For this review, take the finished solid that the model builds, in its own axes (mm). Face numbers are marked on the shaded views. A direction names the side the tool comes from. Coordinates: 2 decimals unless noted, no trailing zeros. Loops run counter-clockwise (first coordinate to the right, second up) from the corner with the lowest first, then second, coordinate; pieces in that order, holes last. Notation, with made-up numbers: (19, 71.5) - (45, 71.5) arc R25 cw to (45, 94.5) - close; hole circle Ø11 at (51, 88.5). An arc over 180 degrees is marked (long way). One line per item, written item: value. Start each with the question number.
1. The part is to be moulded in two halves that separate along X. For the marked faces 3, 4, 5 and 6, say which applies: released by +X, released by -X, zero draft, split by the parting line, or undercut.
2. Insertion check: pin 1 (5.5 mm diameter, centred on x = 0, z = -14, fed in from -Y). The pin has a flat end and moves straight along its axis. Give the tip position at first contact, or say it passes through.
3. To check wall thickness, follow line 1 (Z direction, x = 0, y = 19); line 2 (X direction, y = 21.75, z = 4); line 3 (X direction, y = 10, z = -14). State the ranges of each line that lie inside material, in increasing order. Write a range as from..to.
4. Take a section at B-B, the plane z = -14. State the section outline as (x, y) points, and give its area (3 significant figures).
5. Take a section at D-D, the plane x = 0. State the section outline as (y, z) points, and give its area (3 significant figures).
6. For the marked faces 1 and 2, list the 3-axis set-ups (+Z, -Z, +X, -X, +Y, -Y) from which the entire face can be reached by the end or side of a thin tool; tool diameter is ignored.
7. Take a section at A-A, the plane x = 4.5. State the section outline as (y, z) points.
8. Take a section at C-C, the plane y = 14.5. State the section outline as (x, z) points, and give its area (3 significant figures).
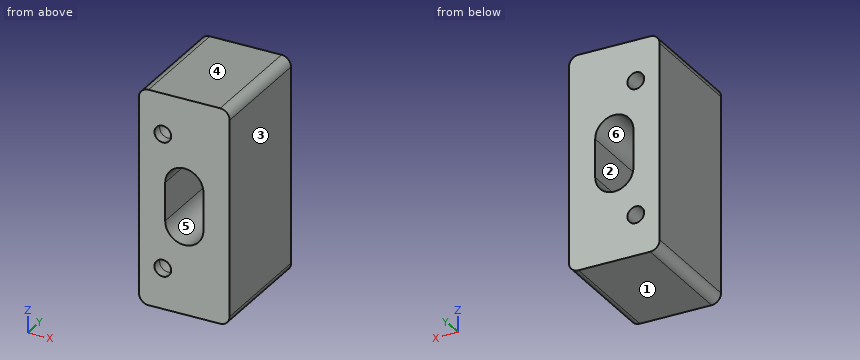
```python
from build123d import *
from build123d.topology import SkipClean

# Parameters (mm, degrees)
SKETCH_1_W          = 19
SKETCH_1_H          = 45
SKETCH_1_R          = 1.75
EXTRUDE_1_DEPTH     = 2
FILLET_1_R          = 2
CUT_EXTRUDE_1_DEPTH = 2
EXTRUDE_START       = 21.612698372
SKETCH_4_R          = 1.75
EXTRUDE_2_DEPTH     = 21.612698372


with BuildPart() as part:
    # 草图1 → 凸台-拉伸1 (new body)
    with BuildSketch(Plane(origin=(0, 0, 0), x_dir=(1, 0, 0), z_dir=(0, 1, 0))):
        with Locations((4.5, 0)):
            Rectangle(SKETCH_1_W, SKETCH_1_H)
        with Locations(Location((0, -14, 0), (0, 0, 270))):
            Circle(SKETCH_1_R, mode=Mode.SUBTRACT)
        with Locations(Location((0, 14, 0), (0, 0, 270))):
            Circle(SKETCH_1_R, mode=Mode.SUBTRACT)
    extrude(amount=EXTRUDE_1_DEPTH)

    # 圆角1
    fillet_1_edges = [part.edges().sort_by_distance(p)[0] for p in [
        (-5, 1, -22.5),
        (14, 1, -22.5),
        (14, 1, 22.5),
        (-5, 1, 22.5),
    ]]
    fillet(fillet_1_edges, radius=FILLET_1_R)

    # 草图3 → 切除-拉伸1 (cut)
    with BuildSketch(Plane(origin=(0, 2, 0), x_dir=(1, 0, 0), z_dir=(0, 1, 0))):
        with BuildLine():
            Line((8.5, 4), (8.5, -4))
            ThreePointArc((8.5, -4), (4.5, -8), (0.5, -4))
            Line((0.5, -4), (0.5, 4))
            ThreePointArc((0.5, 4), (4.5, 8), (8.5, 4))
        make_face()
    extrude(amount=-CUT_EXTRUDE_1_DEPTH, mode=Mode.SUBTRACT)

    # 草图4 → 凸台-拉伸2 (add)
    with SkipClean():  # the faces are left unmerged after this step: merging them gives an invalid solid
        with BuildSketch(Plane(origin=(0, 2, 0), x_dir=(1, 0, 0), z_dir=(0, 1, 0)).offset(EXTRUDE_START)):
            with BuildLine():
                Line((12, 22.5), (-3, 22.5))
                ThreePointArc((-3, 22.5), (-4.414213562, 21.914213562), (-5, 20.5))
                Line((-5, 20.5), (-5, -20.5))
                ThreePointArc((-5, -20.5), (-4.414213562, -21.914213562), (-3, -22.5))
                Line((-3, -22.5), (12, -22.5))
                ThreePointArc((12, -22.5), (13.414213562, -21.914213562), (14, -20.5))
                Line((14, -20.5), (14, 20.5))
                ThreePointArc((14, 20.5), (13.414213562, 21.914213562), (12, 22.5))
            make_face()
            with Locations((0, 14)):
                Circle(SKETCH_4_R, mode=Mode.SUBTRACT)
            with Locations((0, -14)):
                Circle(SKETCH_4_R, mode=Mode.SUBTRACT)
            with BuildLine():
                Line((8.5, -4), (8.5, 4))
                ThreePointArc((8.5, 4), (4.5, 8), (0.5, 4))
                Line((0.5, 4), (0.5, -4))
                ThreePointArc((0.5, -4), (4.5, -8), (8.5, -4))
            make_face(mode=Mode.SUBTRACT)
        extrude(amount=-EXTRUDE_2_DEPTH)
    add(part.part.scale(1), mode=Mode.REPLACE)  # the faces are merged on a copy


solid = part.part
```
Solutions:
1. face 3: released by +X
1. face 4: zero draft
1. face 5: undercut
1. face 6: undercut
2. pin 1: y = 0
3. line 1: -22.5..-15.75, -12.25..12.25, 15.75..22.5
3. line 2: -5..0.5, 8.5..14
3. line 3: -5..-1.75, 1.75..14
4. outline: (-5, 0) - (-1.75, 0) - (-1.75, 23.61) - (-5, 23.61) - close; (1.75, 0) - (14, 0) - (14, 23.61) - (1.75, 23.61) - close
4. area: 366 mm2
5. outline: (0, -22.5) - (23.61, -22.5) - (23.61, -15.75) - (0, -15.75) - close; (0, -12.25) - (23.61, -12.25) - (23.61, 12.25) - (0, 12.25) - close; (0, 15.75) - (23.61, 15.75) - (23.61, 22.5) - (0, 22.5) - close
5. area: 897 mm2
6. face 1: -Z, +X, -X, +Y, -Y
6. face 2: +Y, -Y
7. outline: (0, -22.5) - (23.61, -22.5) - (23.61, -8) - (0, -8) - close; (0, 8) - (23.61, 8) - (23.61, 22.5) - (0, 22.5) - close
8. outline: (-5, -20.5) arc R2 ccw to (-3, -22.5) - (12, -22.5) arc R2 ccw to (14, -20.5) - (14, 20.5) arc R2 ccw to (12, 22.5) - (-3, 22.5) arc R2 ccw to (-5, 20.5) - close; hole circle Ø3.5 at (0, -14); hole circle Ø3.5 at (0, 14); hole (0.5, -4) arc R4 ccw to (8.5, -4) - (8.5, 4) arc R4 ccw to (0.5, 4) - close
8. area: 718 mm2
